Check sheet for the drawn part. Datum: minimum x, y, z corner. Units: mm. A direction names the side the tool comes from. Coordinates: 2 decimals unless noted, no trailing zeros. Order: outer loops, then holes, each group sorted by start corner. A loop starts at its lowest first (then second) coordinate and runs counter-clockwise, first axis right, second up. Notation, with made-up numbers: (64, -16) - (118, -16) arc R36 ccw to (118, 22) - close; hole circle Ø1 at (3.5, 47.25). An arc over 180 degrees is marked (long way). Answer as CSV lines item,"result". Start each with the question number.
1. Material ranges on L1, parallel to Z at x = 34, y = 24; L2, parallel to X at y = 15, z = 18; L3, parallel to X at y = 5.5, z = 17 (1 decimal), recorded low to high. Write a range as [from, to].
2. Mould release check, pull along Z, two halves, no side actions. Record for the marked faces 1, 2 and 3: pulls with the +Z half, pulls with the -Z half, needs draft (parallel to the pull), parting line crosses it, or undercut.
3. Section check A-A (x = 8.5). Record the cut outline in (y, z).
4. Section check B-B (y = 28.5). Record the cut outline in (x, z).
5. Go/stop test with flat-tipped pins: pin 1 (10 mm diameter, centred on y = 12, z = 12.5, fed in from -X); pin 2 (11.5 mm diameter, centred on x = 19, y = 19.5, fed in from +Z) (1 decimal); pin 3 (12 mm diameter, centred on x = 28, y = 18.5, fed in from +Z). Record where each tip stops, or that it passes through.
6. Section check C-C (z = 9.5). Record the cut outline in (x, y) (1 decimal).
7. Section check D-D (x = 46.5). Record the cut outline in (y, z), and give its area (3 significant figures).
8. Set-up check for the marked faces 4 and 5: record each of +Z, -Z, +X, -X, +Y, -Y from which the full face is reachable in a straight line by a thin tool's end or side.
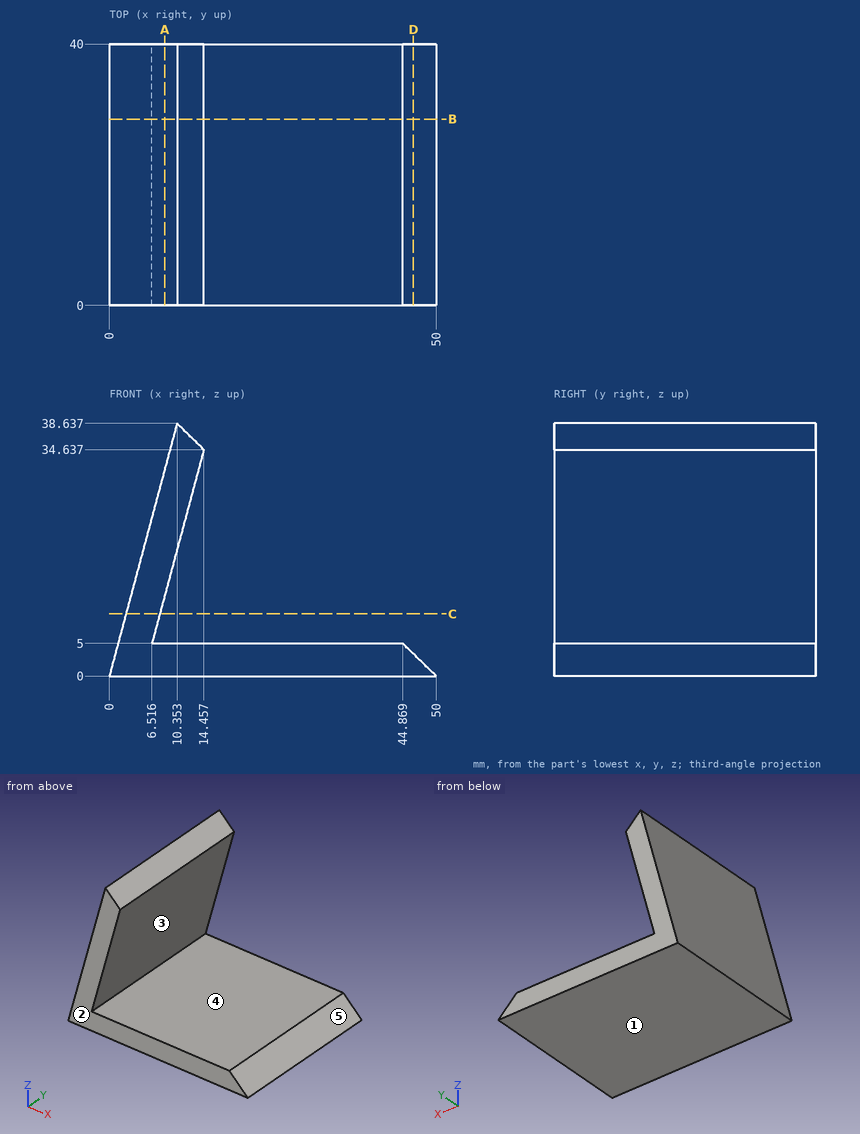
Evaluation:
1,L1,"z = [0, 5]"
1,L2,"x = [4.82, 10]"
1,L3,"x = [4.6, 9.7]"
2,face 1,"pulls with the -Z half"
2,face 2,"needs draft"
2,face 3,"undercut"
3,outline,"(0, 0) - (40, 0) - (40, 5) - (0, 5) - close; (0, 12.4) - (40, 12.4) - (40, 31.72) - (0, 31.72) - close"
4,outline,"(0, 0) - (50, 0) - (44.87, 5) - (6.52, 5) - (14.46, 34.64) - (10.35, 38.64) - close"
5,pin 1,"stops at x = 2.01"
5,pin 2,"stops at z = 35.8"
5,pin 3,"stops at z = 5"
6,outline,"(2.5, 0) - (7.7, 0) - (7.7, 40) - (2.5, 40) - close"
7,outline,"(0, 0) - (40, 0) - (40, 3.41) - (0, 3.41) - close"
7,area,"136 mm²"
8,face 4,"+X, +Y, -Y"
8,face 5,"+Z, +X, +Y, -Y"
